Here's the drawing with two shaded views (mm, measured from the low corner). I have some questions. Give positions to 0.01 mm unless a question says otherwise; leave off trailing zeros. Loops run counter-clockwise (first coordinate to the right, second up) from the corner with the lowest first, then second, coordinate; pieces in that order, holes last. Notation, with made-up numbers: M 44,55 L 68,55 A25 cw 68,79 Z; hole C 17.5,-0.75 d6. An arc over 180 degrees is marked long. Answer in a Markdown table with one row per item. Add a question column.
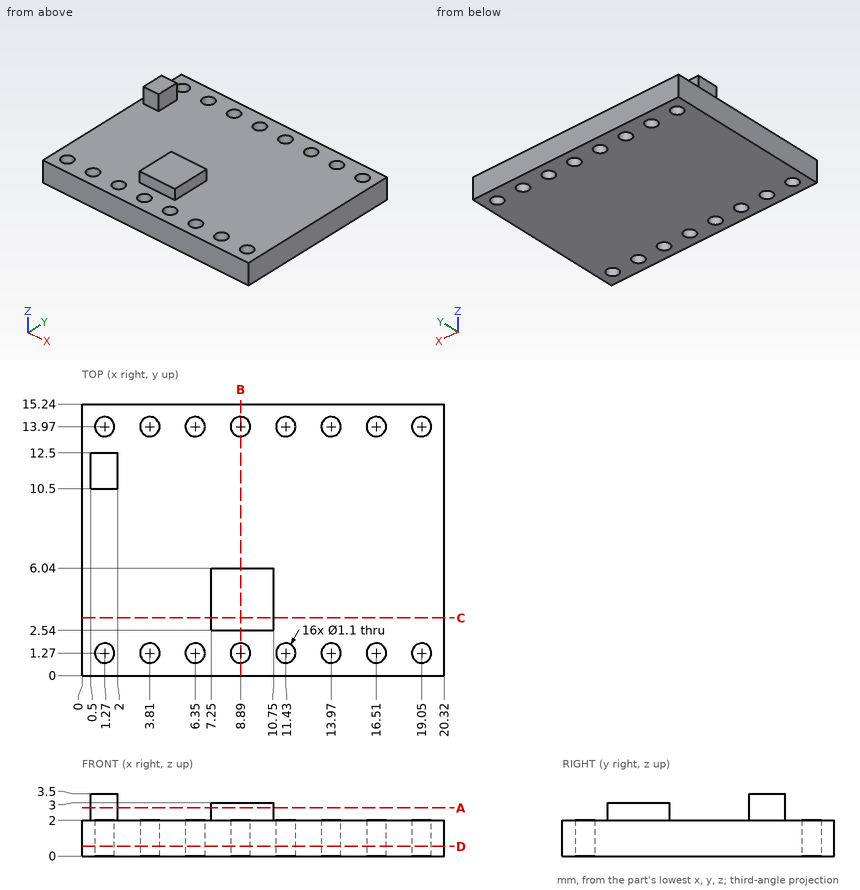
Item 1: For P1, Ø1.1, axis at x = 9.5, z = 2.5, coming from the -Y side; P2, Ø1.4, axis at x = 6.35, y = 1.27, coming from the +Z side; P3, Ø1, axis at y = 10.5, z = 3, coming from the +X side; P4, Ø1.2, axis at x = 1, z = 3, coming from the +Y side, each with a flat end and sliding along its axis, tell me the tip position at first contact or that it passes through.
Item 2: Suppose I cut it at A-A (z = 2.7). List the corners of the cut face in (x, y) for me.
Item 3: I need wall thicknesses on L1, parallel to Y at x = 1.27, z = 0.7; L2, parallel to X at y = 3.25, z = 2.3; L3, parallel to Z at x = 9.5, y = 13.75. Which ranges of each line are inside material? Lowest first, please.
Item 4: Suppose I cut it at C-C (y = 3.25). List the corners of the cut face in (x, z) for me, then the cut area to 3 significant figures.
Item 5: Suppose I cut it at D-D (z = 0.55). Give the number of separate pieces and of enclosed holes in the cut face, then the cut area to 3 significant figures.
Item 6: Suppose I cut it at B-B (x = 8.89). List the corners of the cut face in (y, z) for me, then the cut area to 3 significant figures.
Values found:
| question | item | result |
|---|---|---|
| 1 | P1 | y = 0 |
| 1 | P2 | z = 2 |
| 1 | P3 | x = 2 |
| 1 | P4 | y = 12.5 |
| 2 | outline | M 0.5,10.5 L 2,10.5 L 2,12.5 L 0.5,12.5 Z; M 7.25,2.54 L 10.75,2.54 L 10.75,6.04 L 7.25,6.04 Z |
| 3 | L1 | 0 to 0.72, 1.82 to 13.42, 14.52 to 15.24 |
| 3 | L2 | 7.25 to 10.75 |
| 3 | L3 | 0 to 2 |
| 4 | outline | M 0,0 L 20.32,0 L 20.32,2 L 10.75,2 L 10.75,3 L 7.25,3 L 7.25,2 L 0,2 Z |
| 4 | area | 44.1 mm² |
| 5 | separate pieces | 1 |
| 5 | enclosed holes | 16 |
| 5 | area | 294 mm² |
| 6 | outline | M 0,0 L 0.72,0 L 0.72,2 L 0,2 Z; M 1.82,0 L 13.42,0 L 13.42,2 L 6.04,2 L 6.04,3 L 2.54,3 L 2.54,2 L 1.82,2 Z; M 14.52,0 L 15.24,0 L 15.24,2 L 14.52,2 Z |
| 6 | area | 29.6 mm² |
